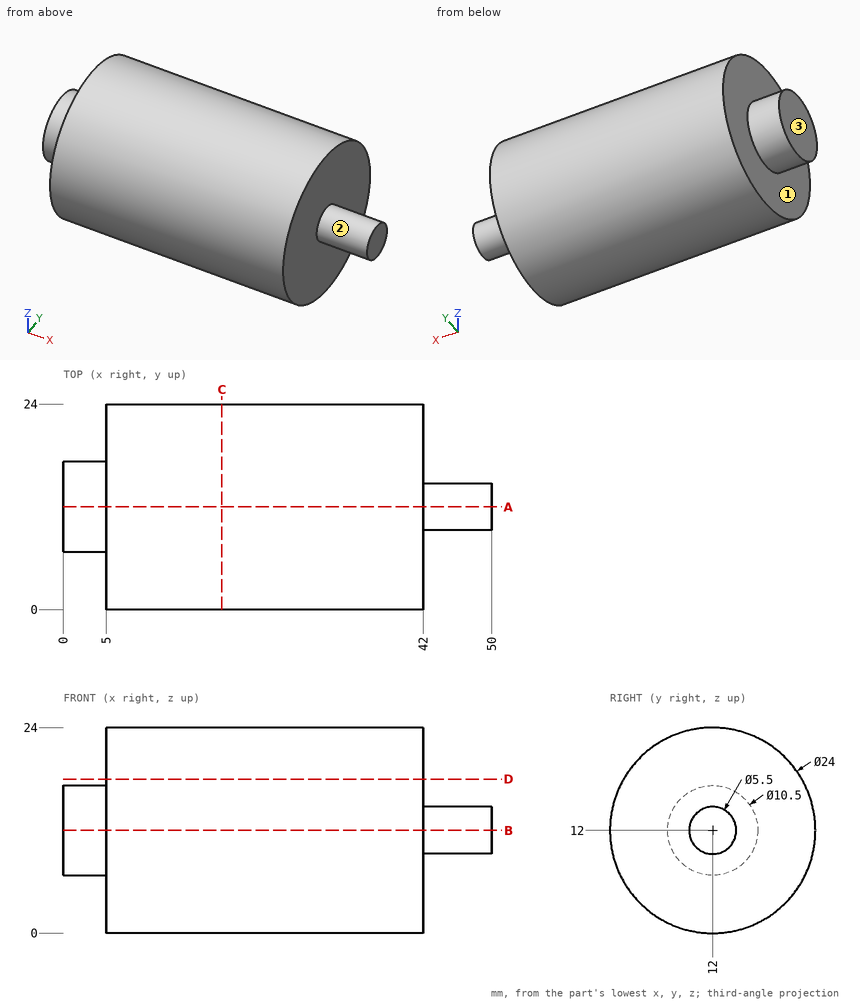
The figure shows three views and two pictorial views of one solid part (mm, origin at its lowest corner). Answer the questions. A direction names the side the tool comes from. Coordinates: 2 decimals unless noted, no trailing zeros. Write each loop counter-clockwise with the first axis right and the second up, starting at its lowest first coordinate (ties: lowest second). Pieces come first, ordered by that corner, then holes. Notation, with made-up numbers: (16, -29) -> (34, -29) arc R26 ccw to (34, 10) -> close; hole circle Ø5 at (60, -31.5). An arc over 180 degrees is marked (long way). Answer as a JSON object with one key per item and string values.
Q1. The part is cut by section D-D on z = 18. Give the vertices of the cut face in (x, y), then the cut area to 3 significant figures.
The answers:
{"outline": "(5, 1.61) -> (42, 1.61) -> (42, 22.39) -> (5, 22.39) -> close", "area": "769 mm2"}
Q2. Consider line 1 (X direction, y = 17, z = 10.5); line 2 (X direction, y = 1.5, z = 10.5); line 3 (Z direction, x = 19, y = 11.5). Determine where each line is inside the solid, lowest interval first. Write a range as [from, to].
The answers:
{"line 1": "x = [0, 42]", "line 2": "x = [5, 42]", "line 3": "z = [0.01, 23.99]"}
Q3. The part is cut by section C-C on x = 18.5. Give the vertices of the cut face in (y, z).
The answers:
{"outline": "circle Ø24 at (12, 12)"}
Q4. Flat-ended cylindrical pins translate along their axes: pin 1 Ø10 at (x, z) = (39, 3.5) entering from -Y; pin 2 Ø1.5 at (x, z) = (6.5, 18.5) entering from +Y; pin 3 Ø6 at (x, z) = (40.5, 18) entering from +Y. Find the tip coordinate at first contact, or state that the pin passes through.
The answers:
{"pin 1": "stops at y = 0.52", "pin 2": "stops at y = 22.53", "pin 3": "stops at y = 23.62"}
Q5. The part is cut by section A-A on y = 12. Give the vertices of the cut face in (x, z), then the cut area to 4 significant figures.
The answers:
{"outline": "(0, 6.75) -> (5, 6.75) -> (5, 0) -> (42, 0) -> (42, 9.25) -> (50, 9.25) -> (50, 14.75) -> (42, 14.75) -> (42, 24) -> (5, 24) -> (5, 17.25) -> (0, 17.25) -> close", "area": "984.5 mm2"}
Q6. A tool of negligible diameter and unlimited length cuts with its end or side. For the marked faces 1, 2 and 3, from which of +Z, -Z, +X, -X, +Y, -Y can it reach the whole face along a straight path? Write none if from no direction.
The answers:
{"face 1": "-X", "face 2": "+X", "face 3": "+Z, -Z, -X, +Y, -Y"}
